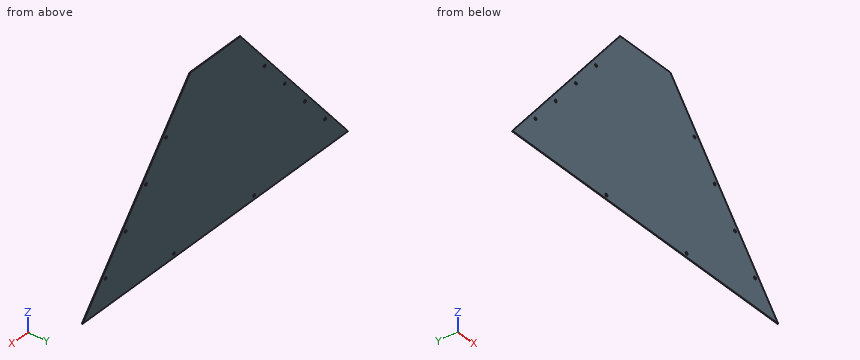
```python
from build123d import *

# Parameters (mm, degrees)
BOSS_EXTRUDE1_DEPTH = 3.175
CUT_EXTRUDE1_REACH  = 5.175
SKETCH2_R           = 6.35
SKETCH4_R           = 6.35
CUT_EXTRUDE2_DEPTH  = 4.175


with BuildPart() as part:
    # Sketch1 → Boss-Extrude1 (new body)
    with BuildSketch(Plane(origin=(0, 0, 0), x_dir=(1, 0, 0), z_dir=(0, 1, 0))):
        Polygon((0, 0), (317.5, 0), (998.5375, 845.729357474), (-681.0375, 845.729357474), align=None)
    extrude(amount=BOSS_EXTRUDE1_DEPTH)

    # Sketch2 → Cut-Extrude1 (cut, up to next)
    with BuildSketch(Plane(origin=(0, 3.175, 0), x_dir=(-1, 0, 0), z_dir=(0, 1, 0)), mode=Mode.PRIVATE) as cut_extrude1_sk1:
        with Locations((87.1855, -826.679357474)):
            Circle(SKETCH2_R)
    cut_extrude1_tool1 = extrude(cut_extrude1_sk1.sketch, amount=-CUT_EXTRUDE1_REACH, mode=Mode.PRIVATE) & part.part
    add(cut_extrude1_tool1.solids().sort_by_distance((-87.1855, 3.175, -826.679357))[0], mode=Mode.SUBTRACT)
    # Sketch2 → Cut-Extrude1 (cut, up to next)
    with BuildSketch(Plane(origin=(0, 3.175, 0), x_dir=(-1, 0, 0), z_dir=(0, 1, 0)), mode=Mode.PRIVATE) as cut_extrude1_sk2:
        with Locations((-420.1795, -826.679357474)):
            Circle(SKETCH2_R)
    cut_extrude1_tool2 = extrude(cut_extrude1_sk2.sketch, amount=-CUT_EXTRUDE1_REACH, mode=Mode.PRIVATE) & part.part
    add(cut_extrude1_tool2.solids().sort_by_distance((420.1795, 3.175, -826.679357))[0], mode=Mode.SUBTRACT)

    # Sketch4 → Cut-Extrude2 (cut, through all)
    with BuildSketch(Plane(origin=(0, 3.175, 0), x_dir=(1, 0, 0), z_dir=(0, 1, 0))):
        with Locations((852.308331977, 704.636230713)):
            Circle(SKETCH4_R)
        with Locations((469.971489871, 229.840801956)):
            Circle(SKETCH4_R)
        with Locations((724.862717941, 546.371087794)):
            Circle(SKETCH4_R)
        with Locations((597.417103906, 388.105944875)):
            Circle(SKETCH4_R)
        with Locations((-534.808331977, 704.636230713)):
            Circle(SKETCH4_R)
        with Locations((-407.362717941, 546.371087794)):
            Circle(SKETCH4_R)
        with Locations((-279.917103906, 388.105944875)):
            Circle(SKETCH4_R)
        with Locations((-152.471489871, 229.840801956)):
            Circle(SKETCH4_R)
    extrude(amount=-CUT_EXTRUDE2_DEPTH, mode=Mode.SUBTRACT)


solid = part.part
```
Work out the finished part from the listing and answer in its coordinate system (mm). Round coordinates to 2 decimals unless told otherwise and drop trailing zeros. Write each loop counter-clockwise with the first axis right and the second up, starting at its lowest first coordinate (ties: lowest second). Pieces come first, ordered by that corner, then holes. Notation, with made-up numbers: (-36.75, 16.25) - (-29.75, 16.25) arc R15 cw to (-29.75, 29.25) - close; hole circle Ø5 at (-2.75, -21.5). An arc over 180 degrees is marked (long way). Return JSON: item names as keys, results as strings. Group by question number.
Q1. The part is cut by section A-A on y = 1.25. Count the separate pieces of the cut face and the enclosed holes in it, then the cut area to 3 significant figures.
Q2. Find the intervals of material crossed by L1, parallel to X at y = 2.6, z = -709; L2, parallel to X at y = 2, z = -546.5; L3, parallel to Z at x = -564.5, y = 2.8, in increasing order.
Q3. This flat-tipped pin is pushed along its axis until it touches: pin 1 Ø3 at (x, z) = (-266.5, -404) entering from -Y. Where does it stop, or does it pass through?
Q4. The part is cut by section C-C on z = -258. Write down the section's boundary in (x, y) (3 decimals).
Q5. The part is cut by section B-B on x = 676. Write down the section's boundary in (y, z) (3 decimals).
Solved:
{
 "1": {"separate pieces": "1", "enclosed holes": "10", "area": "843,000 mm²"},
 "2": {"L1": "-570.93 to -539.42, -530.2 to 847.7, 856.92 to 888.43", "L2": "-440.08 to -413.71, -401.01 to 718.51, 731.21 to 757.58", "L3": "-845.73 to -701.01"},
 "3": {"pin 1": "y = 0"},
 "4": {"outline": "(-207.759, 0) - (525.259, 0) - (525.259, 3.175) - (-207.759, 3.175) - close"},
 "5": {"outline": "(0, -845.729) - (3.175, -845.729) - (3.175, -445.194) - (0, -445.194) - close"}
}
